```python
from build123d import *

# Parameters (mm, degrees)
BOSS_EXTRUDE1_DEPTH = 63.5
SKETCH5_W           = 38.1
SKETCH5_H           = 25.4
CUT_EXTRUDE1_DEPTH  = 19.05
CUT_EXTRUDE2_DEPTH  = 12.7
CUT_EXTRUDE3_DEPTH  = 13.97


with BuildPart() as part:
    # Sketch1 → Boss-Extrude1 (new body)
    with BuildSketch(Plane.XY):
        Polygon((-30.358125429, 24.501905667), (-30.358125429, -24.053030303), (-14.483125429, -24.053030303), (-14.483125429, -12.7), (55.357945402, -12.7), (55.357945402, -25.4), (71.232945402, -25.4), (71.232945402, 0), (7.741874571, 0), (7.741874571, 26.746969697), (-3.41873149, 26.746969697), (-3.41873149, 18.809469697), (-17.658125429, 18.809469697), (-17.658125429, 26.746969697), (-28.113061399, 26.746969697), align=None)
    extrude(amount=BOSS_EXTRUDE1_DEPTH)

    # Sketch5 → Cut-Extrude1 (cut)
    with BuildSketch(Plane(origin=(0, 26.746969697, 0), x_dir=(1, 0, 0), z_dir=(0, 1, 0))):
        with Locations((-11.308125429, -31.75)):
            Rectangle(SKETCH5_W, SKETCH5_H)
    extrude(amount=-CUT_EXTRUDE1_DEPTH, mode=Mode.SUBTRACT)

    # Sketch6 → Cut-Extrude2 (cut)
    with BuildSketch(Plane(origin=(0, 0, 0), x_dir=(1, 0, 0), z_dir=(0, 1, 0))):
        with BuildLine():
            Line((29.459066372, -19.05), (38.786778405, -19.05))
            ThreePointArc((38.786778405, -19.05), (44.46919031, -21.403732078), (46.822922388, -27.086143983))
            Line((46.822922388, -27.086143983), (46.822922388, -36.413856017))
            ThreePointArc((46.822922388, -36.413856017), (44.46919031, -42.096267922), (38.786778405, -44.45))
            Line((38.786778405, -44.45), (29.459066372, -44.45))
            ThreePointArc((29.459066372, -44.45), (23.776654467, -42.096267922), (21.422922388, -36.413856017))
            Line((21.422922388, -36.413856017), (21.422922388, -27.086143983))
            ThreePointArc((21.422922388, -27.086143983), (23.776654467, -21.403732078), (29.459066372, -19.05))
        make_face()
    extrude(amount=-CUT_EXTRUDE2_DEPTH, mode=Mode.SUBTRACT)

    # Sketch7 → Cut-Extrude3 (cut)
    with BuildSketch(Plane(origin=(0, 7.696969697, 0), x_dir=(1, 0, 0), z_dir=(0, 1, 0))):
        with BuildLine():
            Line((-21.28655142, -26.111602122), (-14.029699438, -26.111602122))
            ThreePointArc((-14.029699438, -26.111602122), (-10.982723986, -27.373700678), (-9.720625429, -30.420676131))
            Line((-9.720625429, -30.420676131), (-9.720625429, -33.079323869))
            ThreePointArc((-9.720625429, -33.079323869), (-10.982723986, -36.126299322), (-14.029699438, -37.388397878))
            Line((-14.029699438, -37.388397878), (-21.28655142, -37.388397878))
            ThreePointArc((-21.28655142, -37.388397878), (-24.333526873, -36.126299322), (-25.595625429, -33.079323869))
            Line((-25.595625429, -33.079323869), (-25.595625429, -30.420676131))
            ThreePointArc((-25.595625429, -30.420676131), (-24.333526873, -27.373700678), (-21.28655142, -26.111602122))
        make_face()
    extrude(amount=-CUT_EXTRUDE3_DEPTH, mode=Mode.SUBTRACT)


solid = part.part
```
The model under review builds one solid part; all positions refer to its coordinate system, in mm. A direction names the side the tool comes from. Round coordinates to 2 decimals unless told otherwise and drop trailing zeros. Loops run counter-clockwise (first coordinate to the right, second up) from the corner with the lowest first, then second, coordinate; pieces in that order, holes last. Notation, with made-up numbers: M 47.5,5 L 102.5,5 A12 ccw 102.5,21 Z; hole C -3,64 d9. An arc over 180 degrees is marked long. Put each result on its own line as item: value.
Q1. Consider section B-B, the plane y = -18.5. Give the boundary of the cut face in (x, z), then the cut area to 3 significant figures.
Result set:
outline: M -30.36,0 L -14.48,0 L -14.48,63.5 L -30.36,63.5 Z; M 55.36,0 L 71.23,0 L 71.23,63.5 L 55.36,63.5 Z
area: 2,020 mm²
Q2. Consider section A-A, the plane x = 36.5. Give the boundary of the cut face in (y, z), then the cut area to 3 significant figures.
Result set:
outline: M -12.7,0 L 0,0 L 0,19.05 L -12.7,19.05 Z; M -12.7,44.45 L 0,44.45 L 0,63.5 L -12.7,63.5 Z
area: 484 mm²
Q3. Consider section C-C, the plane z = 40.5. Give the boundary of the cut face in (x, y), then the cut area to 3 significant figures.
Result set:
outline: M -30.36,-24.05 L -14.48,-24.05 L -14.48,-12.7 L 22.54,-12.7 L 22.54,0 L 7.74,0 L 7.74,7.7 L -30.36,7.7 Z; M 45.71,-12.7 L 55.36,-12.7 L 55.36,-25.4 L 71.23,-25.4 L 71.23,0 L 45.71,0 Z
area: 1,670 mm²
Q4. To check wall thickness, follow L1, parallel to Z at x = -21.5, y = 2; L2, parallel to Y at x = 13, z = 47.5; L3, parallel to X at y = 11, z = 6. State the ranges of each line that lie inside material, in increasing order.
Result set:
L1: z = 0 to 26.12, 37.38 to 63.5
L2: y = -12.7 to 0
L3: x = -30.36 to 7.74
Q5. Consider section D-D, the plane y = 1.5. Give the boundary of the cut face in (x, z), then the cut area to 3 significant figures.
Result set:
outline: M -30.36,0 L 7.74,0 L 7.74,63.5 L -30.36,63.5 Z; hole M -25.6,30.42 A4.31 ccw -21.29,26.11 L -14.03,26.11 A4.31 ccw -9.72,30.42 L -9.72,33.08 A4.31 ccw -14.03,37.39 L -21.29,37.39 A4.31 ccw -25.6,33.08 Z
area: 2,260 mm²
Q6. Mouldability with a two-part tool opening along X and no side actions: class faces 6 (the flat face through (-29.22, 25.64, 9.39)), 7 (the flat face through (2, 26.747, 9)), 8 (the flat face through (-10, 18.809, 9)) as released by +X, released by -X, zero draft, split by the parting line, or undercut.
Result set:
face 6: released by -X
face 7: zero draft
face 8: undercut
Q7. For pin 1 (3.5 mm diameter, centred on x = -18.5, y = 1.5, fed in from -Z); pin 2 (3 mm diameter, centred on x = 40, z = 53, fed in from -Y); pin 3 (6.5 mm diameter, centred on y = 21, z = 51, fed in from +X); pin 4 (10 mm diameter, centred on x = 11, z = 33.5, fed in from +Y), all flat-tipped, find the tip position at first contact; note any pin that passes through.
Result set:
pin 1: stops at z = 0
pin 2: stops at y = -12.7
pin 3: stops at x = 7.74
pin 4: stops at y = 7.7
Q8. Machinability: for faces 1 (the flat face through (-14.483, -18, 31)), 2 (the flat face through (-17.658, 23, 9)), 3 (the cylindrical face through (-10.949, 0.81, 36.093)), 4 (the cylindrical face through (23.71, -6.26, 21.47)), 5 (the flat face through (-12, 17, 19.05)), which of the approach directions +Z, -Z, +X, -X, +Y, -Y give a long, thin tool a straight path to every point of the face, cutting with its end or side? Answer none if there is none.
Result set:
face 1: +Z, -Z, -Y
face 2: +Z, -Z, +Y
face 3: +Y
face 4: +Y, -Y
face 5: +X, -X, +Y
